Autodesk Inventor part; units mm, degrees
ref_plane "YZ Plane" through (0, 0, 0) normal (1, 0, 0) x (0, 1, 0)
ref_plane "XZ Plane" through (0, 0, 0) normal (0, 1, 0) x (-1, 0, 0)
ref_plane "XY Plane" through (0, 0, 0) normal (0, 0, 1) x (1, 0, 0)
sketch "Sketch1" plane through (0, 0, 0) normal (0, 0, 1) x (1, 0, 0)
  circle A0 centre (0, 0) radius 7.5 construction
  circle A1 centre (0, 0) radius 4
  arc A2 (0, 7.5) -> (0, -7.5) centre (0, 0) ccw
  line L0 (0, 7.5) -> (50, 7.5)
  line L1 (0, -7.5) -> (50, -7.5)
  circle A3 centre (50, 0) radius 7.5 construction
  arc A4 (50, -7.5) -> (50, 7.5) centre (50, 0) ccw
  circle A5 centre (50, 0) radius 3.5
  dimension "d0" = 15
  dimension "d1" = 8
  dimension "d2" = 50
  dimension "d3" = 7
extrude "Extrusion1" add sketch "Sketch1" along normal blind 10
sketch "Sketch2" plane through (0, 0, 10) normal (0, 0, 1) x (1, 0, 0)
  circle A0 centre (9.4, 0) radius 1.5
  point P0 (0, 0)
  dimension "d6" = 3
  dimension "d7" = 9.4
extrude "Extrusion2" cut sketch "Sketch2" against normal through all
sketch "Sketch3" plane through (0, 0, 10) normal (0, 0, 1) x (1, 0, 0)
  circle A0 centre (9.4, 0) radius 1.5
  circle A1 centre (9.4, 0) radius 3.5
  point P0 (0, 0)
  dimension "d10" = 2
extrude "Extrusion3" cut sketch "Sketch3" against normal blind 3
properties part number "GA004" material "ABS Plastic"
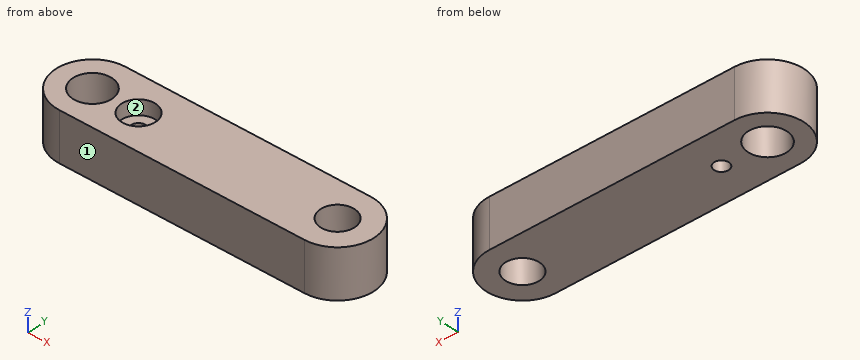
Could you check a few things on this model? Use its own coordinates, in mm. Face numbers are marked on the shaded views. A direction names the side the tool comes from. Give positions to 0.01 mm unless a question says otherwise; leave off trailing zeros. Loops run counter-clockwise (first coordinate to the right, second up) from the corner with the lowest first, then second, coordinate; pieces in that order, holes last. Notation, with made-up numbers: (70.5, 82.5) - (97.5, 82.5) arc R24 ccw to (97.5, 108.5) - close; hole circle Ø3 at (45, -13.5). An arc over 180 degrees is marked (long way). Use one line per item in the form item = value.
1. I want a section at C-C (y = 0). Please give me the cut outline in (x, z).
Response values:
outline = (-7.5, 0) - (-4, 0) - (-4, 10) - (-7.5, 10) - close; (4, 0) - (7.9, 0) - (7.9, 7) - (5.9, 7) - (5.9, 10) - (4, 10) - close; (10.9, 0) - (46.5, 0) - (46.5, 10) - (12.9, 10) - (12.9, 7) - (10.9, 7) - close; (53.5, 0) - (57.5, 0) - (57.5, 10) - (53.5, 10) - close
2. On a 3-axis mill with a long thin cutter (end or side, diameter ignored), from which of +Z, -Z, +X, -X, +Y, -Y can I reach the whole of each face in a straight line? I mean the marked faces 1 and 2. Say none if no direction works.
Response values:
face_1 = +Z, -Z, +X, -X, -Y
face_2 = +Z
3. I want a section at B-B (z = 3.5). Please give me the cut outline in (x, y), and give its area (3 significant figures).
Response values:
outline = (0, -7.5) - (50, -7.5) arc R7.5 ccw to (50, 7.5) - (0, 7.5) arc R7.5 ccw to start; hole circle Ø8 at (0, 0); hole circle Ø3 at (9.4, 0); hole circle Ø7 at (50, 0)
area = 831 mm²
4. I need wall thicknesses on probe 1 along X at (y, z) = (-0.25, 7.25); probe 2 along Y at (x, z) = (9.4, 8); probe 3 along Y at (x, z) = (0, 8.25). Which ranges of each line are inside material? Lowest first, please.
Response values:
probe_1 = -7.5 to -3.99, 3.99 to 5.91, 12.89 to 46.51, 53.49 to 57.5
probe_2 = -7.5 to -3.5, 3.5 to 7.5
probe_3 = -7.5 to -4, 4 to 7.5
5. I want a section at D-D (x = -1). Please give me the cut outline in (y, z), and give its area (3 significant figures).
Response values:
outline = (-7.43, 0) - (-3.87, 0) - (-3.87, 10) - (-7.43, 10) - close; (3.87, 0) - (7.43, 0) - (7.43, 10) - (3.87, 10) - close
area = 71.2 mm²
6. I'm going to push flat-ended pins straight in: pin 1 Ø2 at (y, z) = (5, 3.5) entering from -X; pin 2 Ø6 at (y, z) = (-4.5, 4.5) entering from +X; pin 3 Ø2 at (y, z) = (-4, 9) entering from -X. Where does each tip first touch, or does it pass through?
Response values:
pin_1 = -6.34
pin_2 = 57.35
pin_3 = -6.87
7. I want a section at A-A (x = 9.4). Please give me the cut outline in (y, z).
Response values:
outline = (-7.5, 0) - (-1.5, 0) - (-1.5, 7) - (-3.5, 7) - (-3.5, 10) - (-7.5, 10) - close; (1.5, 0) - (7.5, 0) - (7.5, 10) - (3.5, 10) - (3.5, 7) - (1.5, 7) - close
